```python
from build123d import *

# Parameters (mm, degrees)
F0_W     = 44
F0_H     = 44
F0_W_2   = 40
F0_H_2   = 40
F1_DEPTH = 50
F2_R     = 1.5
F3_DEPTH = 44.001
F4_R     = 2.5
F5_DEPTH = 44.001


with BuildPart() as f1:
    # F0 (on Front) → F1 (new body)
    with BuildSketch(Plane.XZ):
        Rectangle(F0_W, F0_H)
        Rectangle(F0_W_2, F0_H_2, mode=Mode.SUBTRACT)
    extrude(amount=F1_DEPTH)

    # F2 (on face) → F3 (cut, through all)
    with BuildSketch(Plane.XY.offset(22)):
        with Locations((10, -15)):
            Circle(F2_R)
        with Locations((10, -35)):
            Circle(F2_R)
        with Locations((-10, -35)):
            Circle(F2_R)
        with Locations((-10, -15)):
            Circle(F2_R)
    extrude(amount=-F3_DEPTH, mode=Mode.SUBTRACT)

    # F4 (on face) → F5 (cut, through all)
    with BuildSketch(Plane(origin=(-22, 0, 0), x_dir=(0, -1, 0), z_dir=(-1, 0, 0))):
        with Locations((12.5, 0)):
            Circle(F4_R)
        with Locations((27.5, 0)):
            Circle(F4_R)
        with Locations((42.5, 0)):
            Circle(F4_R)
    extrude(amount=-F5_DEPTH, mode=Mode.SUBTRACT)


solid = f1.part
```
Source: CAD feature listing. Evaluate the final solid. Frame: model axes, mm. A direction names the side the tool comes from. Coordinates: 2 decimals unless noted, no trailing zeros. Loops run counter-clockwise (first coordinate to the right, second up) from the corner with the lowest first, then second, coordinate; pieces in that order, holes last. Notation, with made-up numbers: M 48.25,22.25 L 87.25,22.25 A9 ccw 87.25,35.25 Z; hole C 18,-21.75 d4. An arc over 180 degrees is marked long. Put each result on its own line as item: value. Start each with the question number.
1) Contact query for a flat-ended pin moving along its axis: pin 1 Ø3 at (y, z) = (-42.5, 0) entering from -X. Output: stop coordinate, or through.
2) Ray query, L1, parallel to Y at x = -10, z = -21.35; L2, parallel to X at y = -19, z = -16.5. Return the intervals inside material, ascending. Write a range as from..to.
3) Pull-direction query (X, two-part tool) for faces 3 (the face through (-10.325, -36.464, 21.014)), 4 (the face through (-2, -50, -21)), 5 (the face through (-22, -24.6, -0.3)); classes: pulls with the +X half, pulls with the -X half, needs draft (parallel to the pull), parting line crosses it, or undercut.
4) Reachability of faces 1 (the face through (0, -25, 20)), 2 (the face through (0, -25, -22)) from +Z, -Z, +X, -X, +Y, -Y: full face, straight path, thin tool, end or side. Return the list, or none.
5) Cut plane C-C on y = -27.5. Return the cut outline in (x, z).
6) Cut plane B-B on z = -18.5. Return the cut outline in (x, y), then the cut area to 3 significant figures.
7) Cut plane D-D on z = 0. Give the number of separate pieces and of enclosed holes in the cut face, then the cut area to 3 significant figures.
8) Cut plane A-A on x = -4.5. Return the cut outline in (y, z).
The answers:
1. pin 1: passes through
2. L1: y = -50..-36.5, -33.5..-16.5, -13.5..0
2. L2: x = -22..-20, 20..22
3. face 3: undercut
3. face 4: needs draft
3. face 5: pulls with the -X half
4. face 1: +Y, -Y
4. face 2: -Z, +X, -X, +Y, -Y
5. outline: M -22,-22 L 22,-22 L 22,-2.5 L 20,-2.5 L 20,-20 L -20,-20 L -20,-2.5 L -22,-2.5 Z; M -22,2.5 L -20,2.5 L -20,20 L 20,20 L 20,2.5 L 22,2.5 L 22,22 L -22,22 Z
6. outline: M -22,-50 L -20,-50 L -20,0 L -22,0 Z; M 20,-50 L 22,-50 L 22,0 L 20,0 Z
6. area: 200 mm²
7. separate pieces: 8
7. enclosed holes: 0
7. area: 140 mm²
8. outline: M -50,-22 L 0,-22 L 0,-20 L -50,-20 Z; M -50,20 L 0,20 L 0,22 L -50,22 Z
